The listing builds one solid part. Answer for the finished solid, in the listing's coordinates (mm). Face numbers are marked on the shaded views. A direction names the side the tool comes from. Coordinates: 2 decimals unless noted, no trailing zeros. Write each loop counter-clockwise with the first axis right and the second up, starting at its lowest first coordinate (ties: lowest second). Pieces come first, ordered by that corner, then holes. Notation, with made-up numbers: M 18.25,-0.75 L 31.25,-0.75 A27 cw 31.25,24.25 Z; hole C 14,44 d2. An arc over 180 degrees is marked long. Answer as CSV lines item,"result". Start each with the question number.
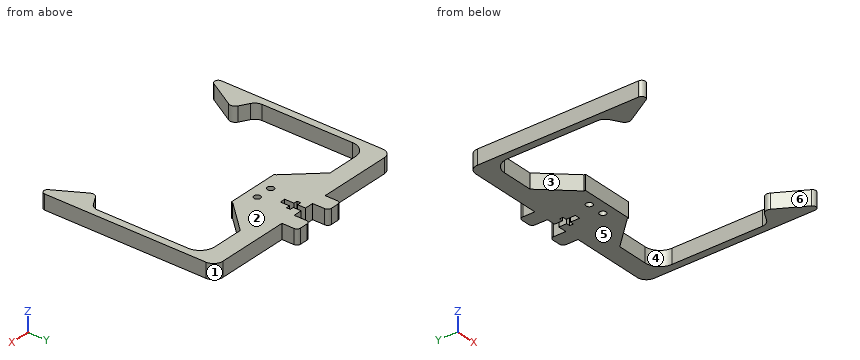
```python
from build123d import *

# Parameters (mm, degrees)
F0_R     = 1.75
F1_DEPTH = 8
F3_DEPTH = 8


with BuildPart() as f1:
    # F0 (on Top) → F1 (new body)
    with BuildSketch(Plane.XY):
        with BuildLine():
            Line((-8.15, -10), (-12.45, -10))
            ThreePointArc((-12.45, -10), (-13.8642135624, -10.5857864376), (-14.45, -12))
            Line((-14.45, -12), (-14.45, -46))
            Line((-14.45, -46), (14.45, -46))
            Line((14.45, -46), (14.45, -12))
            ThreePointArc((14.45, -12), (13.8642135624, -10.5857864376), (12.45, -10))
            Line((12.45, -10), (8.15, -10))
            ThreePointArc((8.15, -10), (6.7357864376, -10.5857864376), (6.15, -12))
            Line((6.15, -12), (6.15, -18.6))
            Line((6.15, -18.6), (1.45, -18.6))
            Line((1.45, -18.6), (1.45, -22.9))
            Line((1.45, -22.9), (3.45, -22.9))
            Line((3.45, -22.9), (3.45, -24.9))
            Line((3.45, -24.9), (1.45, -24.9))
            Line((1.45, -24.9), (1.45, -29.9))
            Line((1.45, -29.9), (-1.45, -29.9))
            Line((-1.45, -29.9), (-1.45, -24.9))
            Line((-1.45, -24.9), (-3.45, -24.9))
            Line((-3.45, -24.9), (-3.45, -22.9))
            Line((-3.45, -22.9), (-1.45, -22.9))
            Line((-1.45, -22.9), (-1.45, -18.6))
            Line((-1.45, -18.6), (-6.15, -18.6))
            Line((-6.15, -18.6), (-6.15, -12))
            ThreePointArc((-6.15, -12), (-6.7357864376, -10.5857864376), (-8.15, -10))
        make_face()
        with Locations((-4.5, -40)):
            Circle(F0_R, mode=Mode.SUBTRACT)
        with Locations((4.5, -40)):
            Circle(F0_R, mode=Mode.SUBTRACT)
    extrude(amount=F1_DEPTH)

    # F2 (on Top) → F3 (join)
    with BuildSketch(Plane.XY):
        with BuildLine():
            Line((-14.2, -45.5), (-10.8380588046, -18.5))
            Line((-10.8380588046, -18.5), (-54, -18.5))
            ThreePointArc((-54, -18.5), (-57.5355339059, -19.9644660941), (-59, -23.5))
            Line((-59, -23.5), (-59, -111.0581123827))
            ThreePointArc((-59, -111.0581123827), (-57.5176380902, -112.9899640353), (-55.2679491924, -112.0581123827))
            Line((-55.2679491924, -112.0581123827), (-46.5, -96.8715789032))
            ThreePointArc((-46.5, -96.8715789032), (-46.2002987325, -94.5951217679), (-47.5980762114, -92.7735026919))
            Line((-47.5980762114, -92.7735026919), (-52.5, -89.943375673))
            ThreePointArc((-52.5, -89.943375673), (-54.3301270189, -88.1132486541), (-55, -85.6132486541))
            Line((-55, -85.6132486541), (-55, -36.5))
            ThreePointArc((-55, -36.5), (-52.6568542495, -30.8431457505), (-47, -28.5))
            Line((-47, -28.5), (-30, -28.5))
            Line((-30, -28.5), (-14.2, -45.5))
        make_face()
    extrude(amount=F3_DEPTH)

    # F4: F1 across plane


with BuildPart() as f1_1:
    add(f1.part)
    add(f1.part.mirror(Plane.YZ))


solid = f1_1.part
```
1) For a pull along X with two mould halves and no side action, classify the marked faces 1, 2, 3 and 4 as +X half, -X half, draft (parallel to the pull), parting line (faces both ways), or undercut.
2) The part is cut by section A-A (y = -50). Determine the outline of the cut face in (x, z), then the cut area to 3 significant figures.
3) Find the intervals of material crossed by line 1 (X direction, y = -71.5, z = 1.25); line 2 (Y direction, x = 4.5, z = 3.75); line 3 (Y direction, x = -35.5, z = 1.25), in increasing order. Write a range as from..to.
4) Each of these flat-tipped pins is pushed along its axis until it touches: P1, Ø1.5, axis at x = 1, z = 6, coming from the -Y side; P2, Ø1.5, axis at x = -41, z = 6, coming from the +Y side; P3, Ø2, axis at y = -21.5, z = 3, coming from the -X side; P4, Ø5.5, axis at x = 4.5, y = -40, coming from the +Z side. Where does it stop, or does it pass through?
5) Which of the six approach directions +Z, -Z, +X, -X, +Y, -Y give full straight-line access (tool end or side, diameter ignored) to the marked faces 5 and 6?
6) The part is cut by section C-C (z = 3.75). Count the separate pieces of the cut face and the enclosed holes in it, then the cut area to 3 significant figures.
7) The part is cut by section D-D (x = -10). Determine the outline of the cut face in (y, z).
8) The part is cut by section B-B (y = -104). Determine the outline of the cut face in (x, z).
Completed:
1,face 1,"+X half"
1,face 2,"draft"
1,face 3,"undercut"
1,face 4,"undercut"
2,outline,"M -59,0 L -55,0 L -55,8 L -59,8 Z; M 55,0 L 59,0 L 59,8 L 55,8 Z"
2,area,"64.0 mm²"
3,line 1,"-59..-55, 55..59"
3,line 2,"-46..-41.75, -38.25..-18.6"
3,line 3,"-28.5..-18.5"
4,P1,"y = -46"
4,P2,"y = -18.5"
4,P3,"x = -58.9"
4,P4,"z = 8"
5,face 5,"-Z, +X, -X, +Y, -Y"
5,face 6,"+Z, -Z, -Y"
6,separate pieces,"1"
6,enclosed holes,"2"
6,area,"2,940 mm²"
7,outline,"M -46,0 L -10,0 L -10,8 L -46,8 Z"
8,outline,"M -59,0 L -50.62,0 L -50.62,8 L -59,8 Z; M 50.62,0 L 59,0 L 59,8 L 50.62,8 Z"
